Input: part model. Units: mm. Frame: model coordinates. A direction names the side the tool comes from. Coordinates: 2 decimals unless noted, no trailing zeros. Loops run counter-clockwise (first coordinate to the right, second up) from the corner with the lowest first, then second, coordinate; pieces in that order, holes last. Notation, with made-up numbers: (-26, -39) - (24, -39) arc R17 cw to (24, -33) - close; hole circle Ø7 at (80.5, 2.25). An arc over 180 degrees is marked (long way). Use one line per item in the form item = value.
from build123d import *

# Parameters (mm, degrees)
SKETCH1_W                      = 152.4
SKETCH1_H                      = 101.6
BASE_FLANGE1_DEPTH             = 1.6002
EDGE_FLANGE1_DEPTH             = 152.4
EDGE_FLANGE2_DEPTH             = 152.4
CUT_EXTRUDE1_DEPTH             = 95.949783169
EDGE_FLANGE7_STRIP_W           = 7.874
EDGE_FLANGE7_STRIP_H           = 1.6002
EDGE_FLANGE7_STRIP_CUT_DEPTH   = 152.4
EDGE_FLANGE7_DEPTH             = 152.4
EDGE_FLANGE8_STRIP_W           = 7.874
EDGE_FLANGE8_STRIP_H           = 1.6002
EDGE_FLANGE8_STRIP_CUT_DEPTH   = 152.4
EDGE_FLANGE8_DEPTH             = 152.4
SKETCH35_W                     = 36.50996
SKETCH35_H                     = 1.6002
BOSS_EXTRUDE1_DEPTH            = 16.0528
EDGE_FLANGE9_STRIP_W           = 7.874
EDGE_FLANGE9_STRIP_H           = 1.6002
EDGE_FLANGE9_STRIP_CUT_DEPTH   = 36.50996
EDGE_FLANGE9_DEPTH             = 36.50996
SKETCH39_W                     = 36.50996
SKETCH39_H                     = 1.6002
BOSS_EXTRUDE2_DEPTH            = 16.0528
EDGE_FLANGE10_STRIP_W          = 7.874
EDGE_FLANGE10_STRIP_H          = 1.6002
EDGE_FLANGE10_STRIP_CUT_DEPTH  = 36.50996
EDGE_FLANGE10_DEPTH            = 36.50996
CUT_EXTRUDE2_REACH             = 114.257
SKETCH43_R                     = 3.37312
CUT_EXTRUDE2_DIRECTION_2_REACH = 114.257
FILLET1_R                      = 12.7
CUT_EXTRUDE3_REACH             = 134.235
SKETCH46_R                     = 5.715


# Sheet-metal steps are written as plain solids
with BuildPart() as part:
    # Sketch1 → Base-Flange1 (new body)
    with BuildSketch(Plane.XY):
        Rectangle(SKETCH1_W, SKETCH1_H)
    extrude(amount=-BASE_FLANGE1_DEPTH)

    # Edge-Flange1 section (across the edge) → Edge-Flange1 (add)
    with BuildSketch(Plane(origin=(-76.2, 51.5366, -1.6002), x_dir=(0, -1, 0), z_dir=(1, 0, 0))):
        with BuildLine():
            Line((-1.6002, 0.7366), (-1.6002, 18.034))
            Line((-1.6002, 18.034), (0, 18.034))
            Line((0, 18.034), (0, 0.7366))
            ThreePointArc((0, 0.7366), (0.215745145, 0.215745145), (0.7366, 0))
            Line((0.7366, 0), (0.7366, -1.6002))
            ThreePointArc((0.7366, -1.6002), (-0.915767126, -0.915767126), (-1.6002, 0.7366))
        make_face()
    extrude(amount=EDGE_FLANGE1_DEPTH)

    # Edge-Flange2 section (across the edge) → Edge-Flange2 (add)
    with BuildSketch(Plane(origin=(76.2, -51.5366, -1.6002), x_dir=(0, 1, 0), z_dir=(-1, 0, 0))):
        with BuildLine():
            Line((-1.6002, 0.7366), (-1.6002, 18.034))
            Line((-1.6002, 18.034), (0, 18.034))
            Line((0, 18.034), (0, 0.7366))
            ThreePointArc((0, 0.7366), (0.215745145, 0.215745145), (0.7366, 0))
            Line((0.7366, 0), (0.7366, -1.6002))
            ThreePointArc((0.7366, -1.6002), (-0.915767126, -0.915767126), (-1.6002, 0.7366))
        make_face()
    extrude(amount=EDGE_FLANGE2_DEPTH)

    # Sketch14 → Cut-Extrude1 (cut, through all)
    with BuildSketch(Plane.XY):
        Polygon((76.2, -38.1), (76.2, 38.1), (38.1, 38.1), (38.1, -16.51), (15.24, -16.51), (15.24, -38.1), align=None)
    extrude(amount=-CUT_EXTRUDE1_DEPTH, mode=Mode.SUBTRACT)

    # Edge-Flange7 strip (across the edge) → Edge-Flange7 strip cut (cut)
    with BuildSketch(Plane(origin=(76.2, -51.5366, -19.6342), x_dir=(0, 0, 1), z_dir=(-1, 0, 0))):
        with Locations((-1.6002, -0.8001)):
            Rectangle(EDGE_FLANGE7_STRIP_W, EDGE_FLANGE7_STRIP_H)
    extrude(amount=EDGE_FLANGE7_STRIP_CUT_DEPTH, mode=Mode.SUBTRACT)

    # Edge-Flange7 section (across the edge) → Edge-Flange7 (add)
    with BuildSketch(Plane(origin=(76.2, -51.5366, -19.6342), x_dir=(0, 0, 1), z_dir=(-1, 0, 0))):
        with BuildLine():
            Line((0, 0.7366), (0, 8.5598))
            Line((0, 8.5598), (1.6002, 8.5598))
            Line((1.6002, 8.5598), (1.6002, 0.7366))
            ThreePointArc((1.6002, 0.7366), (1.815945145, 0.215745145), (2.3368, 0))
            Line((2.3368, 0), (2.3368, -1.6002))
            ThreePointArc((2.3368, -1.6002), (0.684432874, -0.915767126), (0, 0.7366))
        make_face()
    extrude(amount=EDGE_FLANGE7_DEPTH)

    # Edge-Flange8 strip (across the edge) → Edge-Flange8 strip cut (cut)
    with BuildSketch(Plane(origin=(-76.2, 51.5366, -19.6342), x_dir=(0, 0, 1), z_dir=(1, 0, 0))):
        with Locations((-1.6002, -0.8001)):
            Rectangle(EDGE_FLANGE8_STRIP_W, EDGE_FLANGE8_STRIP_H)
    extrude(amount=EDGE_FLANGE8_STRIP_CUT_DEPTH, mode=Mode.SUBTRACT)

    # Edge-Flange8 section (across the edge) → Edge-Flange8 (add)
    with BuildSketch(Plane(origin=(-76.2, 51.5366, -19.6342), x_dir=(0, 0, 1), z_dir=(1, 0, 0))):
        with BuildLine():
            Line((0, 0.7366), (0, 8.5598))
            Line((0, 8.5598), (1.6002, 8.5598))
            Line((1.6002, 8.5598), (1.6002, 0.7366))
            ThreePointArc((1.6002, 0.7366), (1.815945145, 0.215745145), (2.3368, 0))
            Line((2.3368, 0), (2.3368, -1.6002))
            ThreePointArc((2.3368, -1.6002), (0.684432874, -0.915767126), (0, 0.7366))
        make_face()
    extrude(amount=EDGE_FLANGE8_DEPTH)

    # Sketch35 → Boss-Extrude1 (add)
    with BuildSketch(Plane(origin=(0, -42.9768, 0), x_dir=(1, 0, 0), z_dir=(0, 1, 0))):
        with Locations((57.94502, 18.8341)):
            Rectangle(SKETCH35_W, SKETCH35_H)
    extrude(amount=BOSS_EXTRUDE1_DEPTH)

    # Edge-Flange9 strip (across the edge) → Edge-Flange9 strip cut (cut)
    with BuildSketch(Plane(origin=(76.2, -26.924, -18.034), x_dir=(0, -1, 0), z_dir=(-1, 0, 0))):
        with Locations((-1.6002, -0.8001)):
            Rectangle(EDGE_FLANGE9_STRIP_W, EDGE_FLANGE9_STRIP_H)
    extrude(amount=EDGE_FLANGE9_STRIP_CUT_DEPTH, mode=Mode.SUBTRACT)

    # Edge-Flange9 section (across the edge) → Edge-Flange9 (add)
    with BuildSketch(Plane(origin=(76.2, -26.924, -18.034), x_dir=(0, -1, 0), z_dir=(-1, 0, 0))):
        with BuildLine():
            Line((0, 0.7366), (0, 13.6398))
            Line((0, 13.6398), (1.6002, 13.6398))
            Line((1.6002, 13.6398), (1.6002, 0.7366))
            ThreePointArc((1.6002, 0.7366), (1.815945145, 0.215745145), (2.3368, 0))
            Line((2.3368, 0), (2.3368, -1.6002))
            ThreePointArc((2.3368, -1.6002), (0.684432874, -0.915767126), (0, 0.7366))
        make_face()
    extrude(amount=EDGE_FLANGE9_DEPTH)

    # Sketch39 → Boss-Extrude2 (add)
    with BuildSketch(Plane.XZ.offset(-42.9768)):
        with Locations((57.94502, -18.8341)):
            Rectangle(SKETCH39_W, SKETCH39_H)
    extrude(amount=BOSS_EXTRUDE2_DEPTH)

    # Edge-Flange10 strip (across the edge) → Edge-Flange10 strip cut (cut)
    with BuildSketch(Plane(origin=(39.69004, 26.924, -18.034), x_dir=(0, 1, 0), z_dir=(1, 0, 0))):
        with Locations((-1.6002, -0.8001)):
            Rectangle(EDGE_FLANGE10_STRIP_W, EDGE_FLANGE10_STRIP_H)
    extrude(amount=EDGE_FLANGE10_STRIP_CUT_DEPTH, mode=Mode.SUBTRACT)

    # Edge-Flange10 section (across the edge) → Edge-Flange10 (add)
    with BuildSketch(Plane(origin=(39.69004, 26.924, -18.034), x_dir=(0, 1, 0), z_dir=(1, 0, 0))):
        with BuildLine():
            Line((0, 0.7366), (0, 13.6398))
            Line((0, 13.6398), (1.6002, 13.6398))
            Line((1.6002, 13.6398), (1.6002, 0.7366))
            ThreePointArc((1.6002, 0.7366), (1.815945145, 0.215745145), (2.3368, 0))
            Line((2.3368, 0), (2.3368, -1.6002))
            ThreePointArc((2.3368, -1.6002), (0.684432874, -0.915767126), (0, 0.7366))
        make_face()
    extrude(amount=EDGE_FLANGE10_DEPTH)

    # Cut-Extrude2: up to this face of the body (flat: up to its plane)
    cut_extrude2_end = Plane(part.part.faces().sort_by_distance((57.94502, -28.5242, -10.8458))[0])
    # Sketch43 → Cut-Extrude2 (cut, up to the picked face)
    with BuildSketch(Plane(origin=(0, -26.924, 0), x_dir=(1, 0, 0), z_dir=(0, 1, 0)), mode=Mode.PRIVATE) as cut_extrude2_sk1:
        with Locations(Location((57.94502, 10.7442, 0), (0, 0, 270))):
            Circle(SKETCH43_R)
    cut_extrude2_tool1 = split(extrude(cut_extrude2_sk1.sketch, amount=-CUT_EXTRUDE2_REACH, mode=Mode.PRIVATE), bisect_by=cut_extrude2_end, keep=Keep.BOTH, mode=Mode.PRIVATE)
    add(cut_extrude2_tool1.solids().sort_by(Axis((57.94502, -26.924, -10.7442), (0, -1, 0)))[0], mode=Mode.SUBTRACT)

    # Cut-Extrude2 direction 2: up to this face of the body (flat: up to its plane)
    cut_extrude2_direction_2_end = Plane(part.part.faces().sort_by_distance((57.94502, 28.5242, -10.8458))[0])
    # Sketch43 → Cut-Extrude2 direction 2 (cut, up to the picked face)
    with BuildSketch(Plane(origin=(0, -26.924, 0), x_dir=(1, 0, 0), z_dir=(0, 1, 0)), mode=Mode.PRIVATE) as cut_extrude2_direction_2_sk1:
        with Locations(Location((57.94502, 10.7442, 0), (0, 0, 270))):
            Circle(SKETCH43_R)
    cut_extrude2_direction_2_tool1 = split(extrude(cut_extrude2_direction_2_sk1.sketch, amount=CUT_EXTRUDE2_DIRECTION_2_REACH, mode=Mode.PRIVATE), bisect_by=cut_extrude2_direction_2_end, keep=Keep.BOTH, mode=Mode.PRIVATE)
    add(cut_extrude2_direction_2_tool1.solids().sort_by(Axis((57.94502, -26.924, -10.7442), (0, 1, 0)))[0], mode=Mode.SUBTRACT)

    # Fillet1
    fillet1_edges = [part.edges().sort_by_distance(p)[0] for p in [
        (39.69004, -42.9768, -18.8341),
        (39.69004, 42.9768, -18.8341),
    ]]
    fillet(fillet1_edges, radius=FILLET1_R)

    # Sketch46 → Cut-Extrude3 (cut, up to next)
    with BuildSketch(Plane.XZ.offset(53.1368), mode=Mode.PRIVATE) as cut_extrude3_sk1:
        with Locations(Location((57.94502, -10.7442, 0), (0, 0, 270))):
            Circle(SKETCH46_R)
    cut_extrude3_tool1 = extrude(cut_extrude3_sk1.sketch, amount=-CUT_EXTRUDE3_REACH, mode=Mode.PRIVATE) & part.part
    add(cut_extrude3_tool1.solids().sort_by_distance((57.94502, -53.1368, -10.7442))[0], mode=Mode.SUBTRACT)


solid = part.part
Q1. Cut plane C-C, the plane y = -1.5. Return loops of the section in (x, z).
Check values:
outline = (-76.2, -1.6) - (38.1, -1.6) - (38.1, 0) - (-76.2, 0) - close
Q2. Ray query, line 1 along Y through (x, z) = (61.5, -10.25); line 2 along Z through (x, y) = (44, 44); line 3 along Y through (x, z) = (25, -16.75). Return the intervals inside material, ascending. Write a range as [from, to].
Check values:
line_1 = [-28.52, -26.92], [26.92, 28.52], [51.54, 53.14]
line_2 = [-19.63, -18.03], [-1.6, 0]
line_3 = [-53.14, -51.54], [51.54, 53.14]
Q3. Set-up query: faces 5 (the flat face through (62, -26.924, -11)), 6 (the flat face through (39.69, -28, -12)), 7 (the flat face through (16, -45, -18.034)), 8 (the cylindrical face through (35.871, -39.355, -18.845)), 9 (the cylindrical face through (61.29, -27.71, -11.18)). Return all of +Z, -Z, +X, -X, +Y, -Y with unobstructed straight access to the full face (end or side cutting, diameter ignored); none if empty.
Check values:
face_5 = +Z, -Z, +X, -X
face_6 = +Z, -Z, -X
face_7 = +X, -X
face_8 = -Z, -X
face_9 = -Y
Q4. Cut plane D-D, the plane x = 25. Return loops of the section in (y, z).
Check values:
outline = (-53.14, -17.3) arc R2.34 ccw to (-50.8, -19.63) - (-42.98, -19.63) - (-42.98, -18.03) - (-50.8, -18.03) arc R0.74 cw to (-51.54, -17.3) - (-51.54, -2.34) arc R0.74 cw to (-50.8, -1.6) - (-38.1, -1.6) - (-38.1, 0) - (-50.8, 0) arc R2.34 ccw to (-53.14, -2.34) - close; (-16.51, -1.6) - (50.8, -1.6) arc R0.74 cw to (51.54, -2.34) - (51.54, -17.3) arc R0.74 cw to (50.8, -18.03) - (42.98, -18.03) - (42.98, -19.63) - (50.8, -19.63) arc R2.34 ccw to (53.14, -17.3) - (53.14, -2.34) arc R2.34 ccw to (50.8, 0) - (-16.51, 0) - close
Q5. Pull-direction query (X, two-part tool) for faces 1 (the cylindrical face through (36.068, 39.158, -18.823)), 2 (the cylindrical face through (63.61, -52.35, -10)), 3 (the flat face through (62, 28.524, -11)), 4 (the cylindrical face through (61.29, 27.71, -11.18)); classes: pulls with the +X half, pulls with the -X half, needs draft (parallel to the pull), parting line crosses it, or undercut.
Check values:
face_1 = pulls with the -X half
face_2 = undercut
face_3 = needs draft
face_4 = undercut
Q6. Cut plane B-B, the plane x = -45. Return loops of the section in (y, z), then the cut area to 3 significant figures.
Check values:
outline = (-53.14, -17.3) arc R2.34 ccw to (-50.8, -19.63) - (-42.98, -19.63) - (-42.98, -18.03) - (-50.8, -18.03) arc R0.74 cw to (-51.54, -17.3) - (-51.54, -2.34) arc R0.74 cw to (-50.8, -1.6) - (50.8, -1.6) arc R0.74 cw to (51.54, -2.34) - (51.54, -17.3) arc R0.74 cw to (50.8, -18.03) - (42.98, -18.03) - (42.98, -19.63) - (50.8, -19.63) arc R2.34 ccw to (53.14, -17.3) - (53.14, -2.34) arc R2.34 ccw to (50.8, 0) - (-50.8, 0) arc R2.34 ccw to (-53.14, -2.34) - close
area = 251 mm²
Q7. First-contact query: P1, Ø1.3, axis at x = 21, z = -1, coming from the -Y side; P2, Ø1.3, axis at x = -15.5, z = -19, coming from the +Y side; P3, Ø0.5, axis at y = 11.5, z = -0.5, coming from the +X side. Flat tips, straight axial feed; report the tip coordinate or a pass-through.
Check values:
P1 = -53.03
P2 = 52.89
P3 = 38.1
